from build123d import *

# Parameters (mm, degrees)
SKETCH1_W           = 355.6
SKETCH1_H           = 203.2
BOSS_EXTRUDE1_DEPTH = 3.175
SKETCH2_W           = 101.6
SKETCH2_H           = 101.6
CUT_EXTRUDE1_DEPTH  = 4.175
SKETCH4_W           = 25.4
SKETCH4_H           = 3.175
SKETCH4_W_2         = 3.175
SKETCH4_H_2         = 25.4
CUT_EXTRUDE3_DEPTH  = 4.175


with BuildPart() as part:
    # Sketch1 → Boss-Extrude1 (new body)
    with BuildSketch(Plane(origin=(0, 0, 0), x_dir=(1, 0, 0), z_dir=(0, 1, 0))):
        with Locations((177.8, 101.6)):
            Rectangle(SKETCH1_W, SKETCH1_H)
    extrude(amount=BOSS_EXTRUDE1_DEPTH)

    # Sketch2 → Cut-Extrude1 (cut, through all)
    with BuildSketch(Plane(origin=(0, 3.175, 0), x_dir=(1, 0, 0), z_dir=(0, 1, 0))):
        with Locations((177.8, 101.6)):
            Rectangle(SKETCH2_W, SKETCH2_H)
    extrude(amount=-CUT_EXTRUDE1_DEPTH, mode=Mode.SUBTRACT)

    # Sketch4 → Cut-Extrude3 (cut, through all)
    with BuildSketch(Plane(origin=(0, 3.175, 0), x_dir=(1, 0, 0), z_dir=(0, 1, 0))):
        with Locations((88.9, 1.5875)):
            Rectangle(SKETCH4_W, SKETCH4_H)
        with Locations((177.8, 1.5875)):
            Rectangle(SKETCH4_W, SKETCH4_H)
        with Locations((266.7, 1.5875)):
            Rectangle(SKETCH4_W, SKETCH4_H)
        with Locations((266.7, 201.6125)):
            Rectangle(SKETCH4_W, SKETCH4_H)
        with Locations((177.8, 201.6125)):
            Rectangle(SKETCH4_W, SKETCH4_H)
        with Locations((88.9, 201.6125)):
            Rectangle(SKETCH4_W, SKETCH4_H)
        with Locations((1.5875, 152.4)):
            Rectangle(SKETCH4_W_2, SKETCH4_H_2)
        with Locations((1.5875, 50.8)):
            Rectangle(SKETCH4_W_2, SKETCH4_H_2)
        with Locations((354.0125, 50.8)):
            Rectangle(SKETCH4_W_2, SKETCH4_H_2)
        with Locations((354.0125, 152.4)):
            Rectangle(SKETCH4_W_2, SKETCH4_H_2)
    extrude(amount=-CUT_EXTRUDE3_DEPTH, mode=Mode.SUBTRACT)


solid = part.part
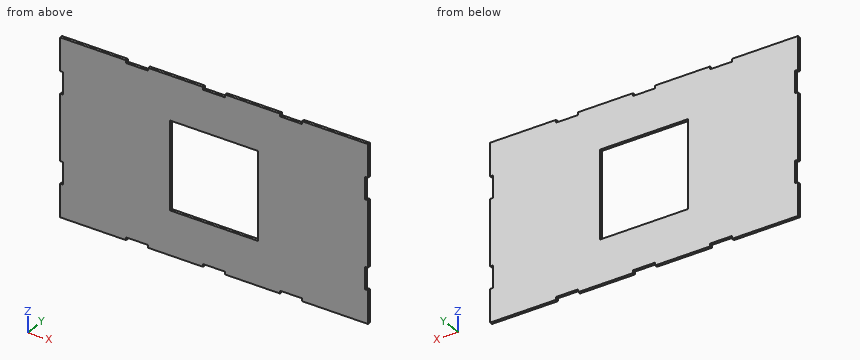
Design review of the part built by this model. Coordinates are the model's own, in mm. Round coordinates to 2 decimals unless told otherwise and drop trailing zeros. Write each loop counter-clockwise with the first axis right and the second up, starting at its lowest first coordinate (ties: lowest second). Pieces come first, ordered by that corner, then holes.
Item 1: Wall thickness on L1, parallel to X at y = 1.5, z = -87; L2, parallel to Z at x = 144, y = 1.2; L3, parallel to X at y = 0.2, z = -62.5 (3 decimals): over which ranges is each line inside the solid? List them lowest first.
Item 2: Consider section B-B on z = -88.5. Give the boundary of the cut face in (x, y) (3 decimals), and give its area (3 significant figures).
Item 3: Consider section D-D on z = -160.5. Give the boundary of the cut face in (x, y) (3 decimals).
Item 4: Consider section A-A on x = 203.5. Give the boundary of the cut face in (y, z) (3 decimals).
Item 5: For pin 1 Ø1.6 at (y, z) = (1, -47) entering from +X (3 decimals); pin 2 Ø1 at (x, y) = (168.5, 1.5) entering from -Z (3 decimals); pin 3 Ø1.6 at (y, z) = (1, -155) entering from -X (3 decimals), all flat-tipped, find the tip position at first contact; note any pin that passes through.
Item 6: Consider section C-C on x = 259.5. Give the boundary of the cut face in (y, z) (3 decimals).
Check values:
1. L1: x = 0 to 127, 228.6 to 355.6
1. L2: z = -203.2 to -152.4, -50.8 to 0
1. L3: x = 3.175 to 127, 228.6 to 352.425
2. outline: (0, 0) - (127, 0) - (127, 3.175) - (0, 3.175) - close; (228.6, 0) - (355.6, 0) - (355.6, 3.175) - (228.6, 3.175) - close
2. area: 806 mm2
3. outline: (3.175, 0) - (352.425, 0) - (352.425, 3.175) - (3.175, 3.175) - close
4. outline: (0, -203.2) - (3.175, -203.2) - (3.175, -152.4) - (0, -152.4) - close; (0, -50.8) - (3.175, -50.8) - (3.175, 0) - (0, 0) - close
5. pin 1: stops at x = 352.425
5. pin 2: stops at z = -200.025
5. pin 3: stops at x = 3.175
6. outline: (0, -200.025) - (3.175, -200.025) - (3.175, -3.175) - (0, -3.175) - close
